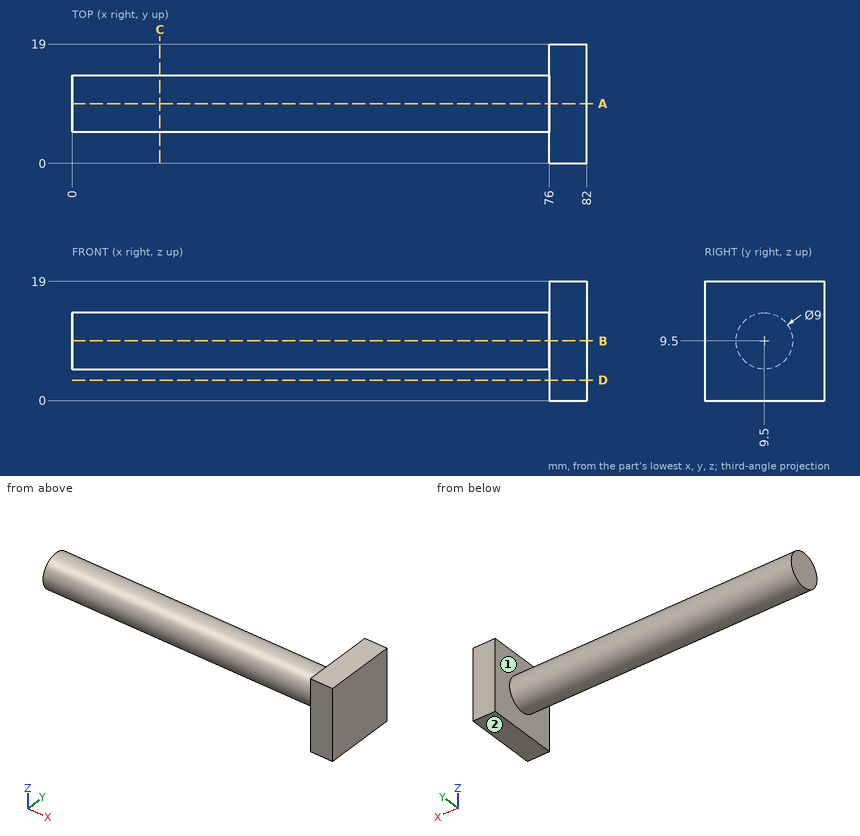
Could you check a few things on this drawing? It's one solid part, dimensions in mm from its lowest x, y, z. A direction names the side the tool comes from. Give positions to 0.01 mm unless a question says otherwise; leave off trailing zeros. Order: outer loops, then holes, each group sorted by start corner. A loop starts at its lowest first (then second) coordinate and runs counter-clockwise, first axis right, second up. Notation, with made-up numbers: (77.5, 23) -> (120.5, 23) arc R18 cw to (120.5, 33) -> close; hole circle Ø5 at (78.5, 55). An arc over 180 degrees is marked (long way). Use CSV: the item, a comma, the result in double quotes. Start each with the question number.
Item 1: Suppose I cut it at C-C (x = 14). List the corners of the cut face in (y, z) for me, and give its area (3 significant figures).
Item 2: I'm going to push flat-ended pins straight in: P1, Ø2, axis at x = 46.5, y = 6.5, coming from the -Z side; P2, Ø6, axis at x = 28.5, y = 7.5, coming from the +Z side; P3, Ø2, axis at x = 9.5, z = 16.5, coming from the -Y side; P4, Ø1, axis at x = 27.5, z = 6, coming from the +Y side. Where does each tip first touch, or does it pass through?
Item 3: Suppose I cut it at A-A (y = 9.5). List the corners of the cut face in (x, z) for me, and give its area (3 significant figures).
Item 4: If I drill on probe 1 along X at (y, z) = (16.25, 7); probe 2 along Y at (x, z) = (32.5, 6); probe 3 along Y at (x, z) = (26, 6.75), over which ranges is the centre line in solid material (lowest first)? Write a range as [from, to].
Item 5: Suppose I cut it at D-D (z = 3.25). List the corners of the cut face in (x, y) for me, and give its area (3 significant figures).
Item 6: On a 3-axis mill with a long thin cutter (end or side, diameter ignored), from which of +Z, -Z, +X, -X, +Y, -Y can I reach the whole of each face in a straight line? I mean the marked faces 1 and 2. Say none if no direction works.
Answer block:
1,outline,"circle Ø9 at (9.5, 9.5)"
1,area,"63.6 mm^2"
2,P1,"stops at z = 5.47"
2,P2,"stops at z = 14"
2,P3,"passes through"
2,P4,"stops at y = 12.85"
3,outline,"(0, 5) -> (76, 5) -> (76, 0) -> (82, 0) -> (82, 19) -> (76, 19) -> (76, 14) -> (0, 14) -> close"
3,area,"798 mm^2"
4,probe 1,"x = [76, 82]"
4,probe 2,"y = [6.67, 12.33]"
4,probe 3,"y = [5.94, 13.06]"
5,outline,"(76, 0) -> (82, 0) -> (82, 19) -> (76, 19) -> close"
5,area,"114 mm^2"
6,face 1,"-X"
6,face 2,"-Z, +X, -X, +Y, -Y"
